The model under review builds one solid part; all positions refer to its coordinate system, in mm. A direction names the side the tool comes from. Round coordinates to 2 decimals unless told otherwise and drop trailing zeros. Write each loop counter-clockwise with the first axis right and the second up, starting at its lowest first coordinate (ties: lowest second). Pieces come first, ordered by that corner, then holes. Notation, with made-up numbers: (60.5, 77.5) - (106.5, 77.5) arc R8 cw to (106.5, 91.5) - close; hole circle Ø3 at (29.25, 27.5). An arc over 180 degrees is marked (long way). Return JSON: item names as keys, results as strings.
from build123d import *

# Parameters (mm, degrees)
SKETCH1_W               = 120
SKETCH1_H               = 45
BOSS_EXTRUDE1_DEPTH     = 12.5
SKETCH3_R               = 2.5
SKETCH3_R_2             = 1.5
BOSS_EXTRUDE2_DEPTH     = 140
SWEEP_THIN2_PROFILE_R   = 2.5
SWEEP_THIN2_PROFILE_R_2 = 1.5
SKETCH53_W              = 80
SKETCH53_H              = 17
BOSS_EXTRUDE3_DEPTH     = 2
SKETCH54_R              = 3.5
BOSS_EXTRUDE4_DEPTH     = 4
LPATTERN1_COUNT         = 2
LPATTERN1_PITCH         = 20
LPATTERN1_COL_COUNT     = 3
LPATTERN1_COL_PITCH     = 20


with BuildPart() as part:
    # Sketch1 → Boss-Extrude1 (new, symmetric)
    with BuildSketch(Plane(origin=(0, 0, 0), x_dir=(1, 0, 0), z_dir=(0, 1, 0))):
        Rectangle(SKETCH1_W, SKETCH1_H)
    extrude(amount=BOSS_EXTRUDE1_DEPTH, both=True)

    # Sketch3 → Boss-Extrude2 (add)
    with BuildSketch(Plane(origin=(0, 12.5, 0), x_dir=(1, 0, 0), z_dir=(0, 1, 0))):
        with Locations(Location((50, 0, 0), (0, 0, 270))):
            Circle(SKETCH3_R)
        with Locations(Location((50, 0, 0), (0, 0, 270))):
            Circle(SKETCH3_R_2, mode=Mode.SUBTRACT)
    extrude(amount=BOSS_EXTRUDE2_DEPTH)

    # Sweep-Thin2: sweep along a path in Sketch57
    with BuildLine(Plane(origin=(0, 0, 0), x_dir=(1, 0, 0), z_dir=(0, 1, 0))) as sweep_thin2_path:
        Line((-60, 13.5), (-113.472065941, 13.5))
        ThreePointArc((-113.472065941, 13.5), (-126.972065941, 0), (-113.472065941, -13.5))
        Line((-113.472065941, -13.5), (-60, -13.5))
    # Sweep-Thin2 profile (on start of the path) → Sweep-Thin2 (sweep)
    with BuildSketch(Plane(origin=(-60, 0, -13.5), x_dir=(0, 0, -1), z_dir=(-1, 0, 0))):
        Circle(SWEEP_THIN2_PROFILE_R)
        Circle(SWEEP_THIN2_PROFILE_R_2, mode=Mode.SUBTRACT)
    sweep(path=sweep_thin2_path.line)

    # Sketch53 → Boss-Extrude3 (add)
    with BuildSketch(Plane.XY.offset(22.5)):
        Rectangle(SKETCH53_W, SKETCH53_H)
    extrude(amount=BOSS_EXTRUDE3_DEPTH)

    # Sketch54 → Boss-Extrude4 (add)
    with BuildSketch(Plane.XY.offset(24.5)):
        with Locations((-10, 0)):
            Circle(SKETCH54_R)
    boss_extrude4 = extrude(amount=BOSS_EXTRUDE4_DEPTH)

    # LPattern1: Boss-Extrude4 ×2
    with Locations(*[(-i * LPATTERN1_PITCH, 0, 0) for i in range(1, LPATTERN1_COUNT)]):
        add(boss_extrude4)

    # LPattern1 col: Boss-Extrude4 ×3
    with Locations(*[(i * LPATTERN1_COL_PITCH, 0, 0) for i in range(1, LPATTERN1_COL_COUNT)]):
        add(boss_extrude4)


solid = part.part
(1) Clearance check with flat-ended pins moving along their axes: pin 1 Ø4 at (y, z) = (9, -7) entering from -X; pin 2 Ø8 at (x, z) = (1.5, 0) entering from +Y; pin 3 Ø1 at (y, z) = (1.5, 23.5) entering from +X; pin 4 Ø8 at (y, z) = (86.5, 9.5) entering from +X. State where each tip first meets the part, or that it passes through.
Filled in:
{"pin 1": "stops at x = -60", "pin 2": "stops at y = 12.5", "pin 3": "stops at x = 40", "pin 4": "passes through"}
(2) Add section C-C (x = -30). Write out the cut boundary in (y, z).
Filled in:
{"outline": "(-12.5, -22.5) - (12.5, -22.5) - (12.5, 22.5) - (8.5, 22.5) - (8.5, 24.5) - (3.5, 24.5) - (3.5, 28.5) - (-3.5, 28.5) - (-3.5, 24.5) - (-8.5, 24.5) - (-8.5, 22.5) - (-12.5, 22.5) - close"}
(3) Add section D-D (z = 20). Write out the cut boundary in (x, y).
Filled in:
{"outline": "(-60, -12.5) - (60, -12.5) - (60, 12.5) - (-60, 12.5) - close"}
(4) Mouldability with a two-part tool opening along X and no side actions: class faces 1 (the flat face through (-1, 12.5, 0)), 2 (the flat face through (60, 0, 0)), 3 (the cylindrical face through (6.503, 0.154, 26.472)) as released by +X, released by -X, zero draft, split by the parting line, or undercut.
Filled in:
{"face 1": "zero draft", "face 2": "released by +X", "face 3": "undercut"}
(5) Add section B-B (y = 111). Write out the cut boundary in (x, z), plus the area to 3 significant figures.
Filled in:
{"outline": "circle Ø5 at (50, 0); hole circle Ø3 at (50, 0)", "area": "12.6 mm2"}
(6) For faces 4 (the cylindrical face through (33.34, 1.05, 26.47)), 5 (the flat face through (30, 0, 28.5)), 6 (the cylindrical face through (-87, 0, -11)), list the 3-axis set-ups (+Z, -Z, +X, -X, +Y, -Y) from which the entire face can be reached by the end or side of a thin tool; tool diameter is ignored.
Filled in:
{"face 4": "+Z", "face 5": "+Z, +X, -X, +Y, -Y", "face 6": "none"}
(7) Wall thickness on line 1 (X direction, y = 77, z = 0); line 2 (Z direction, x = -83, y = 0); line 3 (Y direction, x = -78, z = 13.5): over which ranges is each line inside the solid? List them lowest first.
Filled in:
{"line 1": "x = 47.5 to 48.5, 51.5 to 52.5", "line 2": "z = -16 to -15, -12 to -11, 11 to 12, 15 to 16", "line 3": "y = -2.5 to -1.5, 1.5 to 2.5"}
(8) Add section A-A (x = -67). Write out the cut boundary in (y, z), plus the area to 3 significant figures.
Filled in:
{"outline": "circle Ø5 at (0, -13.5); circle Ø5 at (0, 13.5); hole circle Ø3 at (0, -13.5); hole circle Ø3 at (0, 13.5)", "area": "25.1 mm2"}
